```python
from build123d import *

# Parameters (mm, degrees)
F1_DEPTH = 1.2
F2_DEPTH = 14
F3_R     = 2.5
F4_R     = 3
F4_R_2   = 1.375
F5_DEPTH = 2


with BuildPart() as f1:
    # F0 (on Top) → F1 (new body)
    with BuildSketch(Plane.XY):
        with BuildLine():
            Line((179.464314, 27.344292), (-13.535686, 27.344292))
            Line((-13.535686, 27.344292), (-13.535686, -82.395708))
            ThreePointArc((-13.535686, -82.395708), (-11.233546, -87.953567), (-5.675686, -90.255708))
            Line((-5.675686, -90.255708), (171.604314, -90.255708))
            ThreePointArc((171.604314, -90.255708), (177.162173, -87.953567), (179.464314, -82.395708))
            Line((179.464314, -82.395708), (179.464314, 27.344292))
        make_face()
    extrude(amount=F1_DEPTH)

    # F0 (on Top) → F2 (join)
    with BuildSketch(Plane.XY):
        with BuildLine():
            Line((180.664314, 28.544292), (-14.735686, 28.544292))
            Line((-14.735686, 28.544292), (-14.735686, -82.395708))
            ThreePointArc((-14.735686, -82.395708), (-12.082074, -88.802096), (-5.675686, -91.455708))
            Line((-5.675686, -91.455708), (171.604314, -91.455708))
            ThreePointArc((171.604314, -91.455708), (178.010701, -88.802096), (180.664314, -82.395708))
            Line((180.664314, -82.395708), (180.664314, 28.544292))
        make_face()
        with BuildLine():
            Line((-13.535686, -82.395708), (-13.535686, 27.344292))
            Line((-13.535686, 27.344292), (179.464314, 27.344292))
            Line((179.464314, 27.344292), (179.464314, -82.395708))
            ThreePointArc((179.464314, -82.395708), (177.162173, -87.953567), (171.604314, -90.255708))
            Line((171.604314, -90.255708), (-5.675686, -90.255708))
            ThreePointArc((-5.675686, -90.255708), (-11.233546, -87.953567), (-13.535686, -82.395708))
        make_face(mode=Mode.SUBTRACT)
    extrude(amount=F2_DEPTH)

    # F3
    f3_edges = [f1.edges().sort_by_distance(p)[0] for p in [
        (-14.735686, 28.544292, 7),
        (180.664314, 28.544292, 7),
    ]]
    fillet(f3_edges, radius=F3_R)

    # F4 (on face) → F5 (join)
    with BuildSketch(Plane.XY.offset(1.2)):
        with Locations((-3.247979, -36.737969)):
            Circle(F4_R)
        with Locations((-3.247979, -36.737969)):
            Circle(F4_R_2, mode=Mode.SUBTRACT)
        with Locations((54.752021, -36.737969)):
            Circle(F4_R)
        with Locations((54.752021, -36.737969)):
            Circle(F4_R_2, mode=Mode.SUBTRACT)
        with Locations((54.752021, 12.262031)):
            Circle(F4_R)
        with Locations((54.752021, 12.262031)):
            Circle(F4_R_2, mode=Mode.SUBTRACT)
        with Locations((-3.247979, 12.262031)):
            Circle(F4_R)
        with Locations((-3.247979, 12.262031)):
            Circle(F4_R_2, mode=Mode.SUBTRACT)
    extrude(amount=F5_DEPTH)


solid = f1.part
```
For this review, take the finished solid that the model builds, in its own axes (mm). A direction names the side the tool comes from. Round coordinates to 2 decimals unless told otherwise and drop trailing zeros. Loops run counter-clockwise (first coordinate to the right, second up) from the corner with the lowest first, then second, coordinate; pieces in that order, holes last.
(1) Tool access review of faces 5 (the flat face through (82, -31, 0)), 6 (the flat face through (53, -37, 3.2)): name each direction out of +Z, -Z, +X, -X, +Y, -Y from which nothing blocks a thin tool from reaching the whole face with its end or side.
Returned:
face 5: -Z, +X, -X, +Y, -Y
face 6: +Z
(2) We need section A-A (y = -31). Give the boundary of the cut face in (x, z), plus the area to 3 significant figures.
Returned:
outline: (-14.74, 0) - (180.66, 0) - (180.66, 14) - (179.46, 14) - (179.46, 1.2) - (-13.54, 1.2) - (-13.54, 14) - (-14.74, 14) - close
area: 265 mm2
(3) We need section C-C (x = 65). Give the boundary of the cut face in (y, z), plus the area to 3 significant figures.
Returned:
outline: (-91.46, 0) - (28.54, 0) - (28.54, 14) - (27.34, 14) - (27.34, 1.2) - (-90.26, 1.2) - (-90.26, 14) - (-91.46, 14) - close
area: 175 mm2
(4) Mouldability with a two-part tool opening along X and no side actions: class faces 1 (the cylindrical face through (-12.152, -88.731, 6.902)), 2 (the flat face through (84, 28.544, 7)), 3 (the flat face through (-3, 14, 3.2)), 4 (the flat face through (-5, -37, 3.2)) as released by +X, released by -X, zero draft, split by the parting line, or undercut.
Returned:
face 1: released by -X
face 2: zero draft
face 3: undercut
face 4: undercut
(5) We need section B-B (z = 8). Give the boundary of the cut face in (x, y), plus the area to 3 significant figures.
Returned:
outline: (-14.74, -82.4) arc R9.06 ccw to (-5.68, -91.46) - (171.6, -91.46) arc R9.06 ccw to (180.66, -82.4) - (180.66, 26.04) arc R2.5 ccw to (178.16, 28.54) - (-12.24, 28.54) arc R2.5 ccw to (-14.74, 26.04) - close; hole (-13.54, -82.4) arc R7.86 ccw to (-5.68, -90.26) - (171.6, -90.26) arc R7.86 ccw to (179.46, -82.4) - (179.46, 27.34) - (-13.54, 27.34) - close
area: 740 mm2
(6) Wall thickness on line 1 along Y through (x, z) = (159, 9.25); line 2 along X through (y, z) = (-76.5, 5.5); line 3 along Z through (x, y) = (40, -54.5): over which ranges is each line inside the solid? List them lowest first.
Returned:
line 1: y = -91.46 to -90.26, 27.34 to 28.54
line 2: x = -14.74 to -13.54, 179.46 to 180.66
line 3: z = 0 to 1.2
(7) Clearance check with flat-ended pins moving along their axes: P1, Ø2, axis at x = 55, y = -37.5, coming from the +Z side; P2, Ø1.8, axis at x = 55, y = -36.5, coming from the +Z side. State where each tip first meets the part, or that it passes through.
Returned:
P1: stops at z = 3.2
P2: stops at z = 1.2
